Design review of the part shown in the three views and the two pictorial views. Dimensions are in mm from the part's minimum x, y and z. A direction names the side the tool comes from. Round coordinates to 2 decimals unless told otherwise and drop trailing zeros. Order: outer loops, then holes, each group sorted by start corner. A loop starts at its lowest first (then second) coordinate and runs counter-clockwise, first axis right, second up. Notation, with made-up numbers: (27.5, 6.25) - (73.5, 6.25) arc R22 cw to (73.5, 36.25) - close; hole circle Ø9 at (70, 64.5). An arc over 180 degrees is marked (long way). One line per item, written item: value.
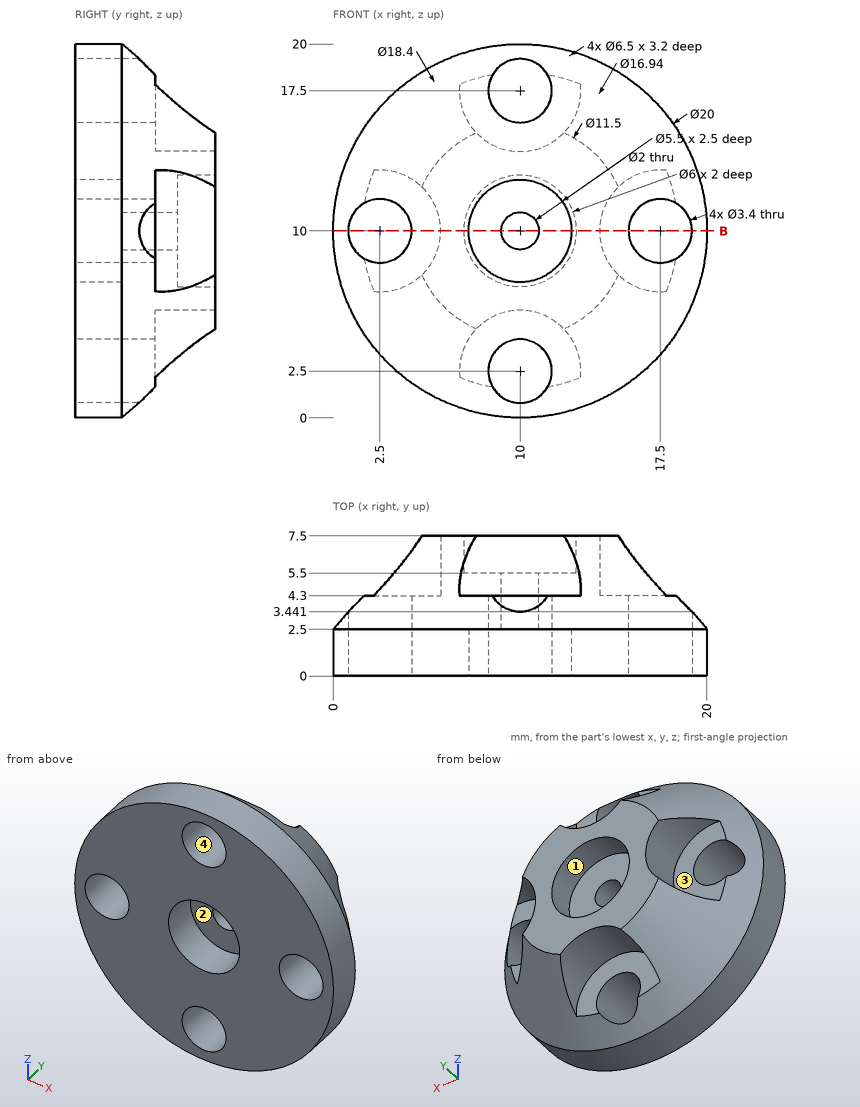
Item 1: Take a section at B-B (z = 10). Write out the cut boundary in (x, y), plus the area to 3 significant figures.
Returned:
outline: (0, 0) - (0.8, 0) - (0.8, 3.44) - (0, 2.5) - close; (4.2, 0) - (7.25, 0) - (7.25, 2.5) - (9, 2.5) - (9, 5.5) - (7, 5.5) - (7, 7.5) - (5.75, 7.5) - (5.75, 4.3) - (4.2, 4.3) - close; (11, 2.5) - (12.75, 2.5) - (12.75, 0) - (15.8, 0) - (15.8, 4.3) - (14.25, 4.3) - (14.25, 7.5) - (13, 7.5) - (13, 5.5) - (11, 5.5) - close; (19.2, 0) - (20, 0) - (20, 2.5) - (19.2, 3.44) - close
area: 50.1 mm^2
Item 2: Machinability: for the marked faces 1, 2, 3 and 4, which of the approach directions +Z, -Z, +X, -X, +Y, -Y give a long, thin tool a straight path to every point of the face, cutting with its end or side? Answer none if there is none.
Returned:
face 1: +Y
face 2: -Y
face 3: -X, +Y
face 4: +Y, -Y
Item 3: For P1, Ø4, axis at x = 10, z = 17.5, coming from the +Y side; P2, Ø4.5, axis at x = 10, z = 10, coming from the +Y side; P3, Ø1.6, axis at x = 9, z = 8.5, coming from the -Y side, all flat-tipped, find the tip position at first contact; note any pin that passes through.
Returned:
P1: y = 4.3
P2: y = 5.5
P3: y = 2.5
Item 4: Wall thickness on line 1 (Z direction, x = 9.25, y = 1.5) (1 decimal); line 2 (Z direction, x = 11.5, y = 1.5) (1 decimal); line 3 (Y direction, x = 15.75, z = 8): over which ranges is each line inside the solid? List them lowest first.
Returned:
line 1: 0 to 1, 4 to 7.4, 12.6 to 16, 19 to 20
line 2: 0.1 to 1.7, 3.3 to 7.7, 12.3 to 16.7, 18.3 to 19.9
line 3: 0 to 4.3
